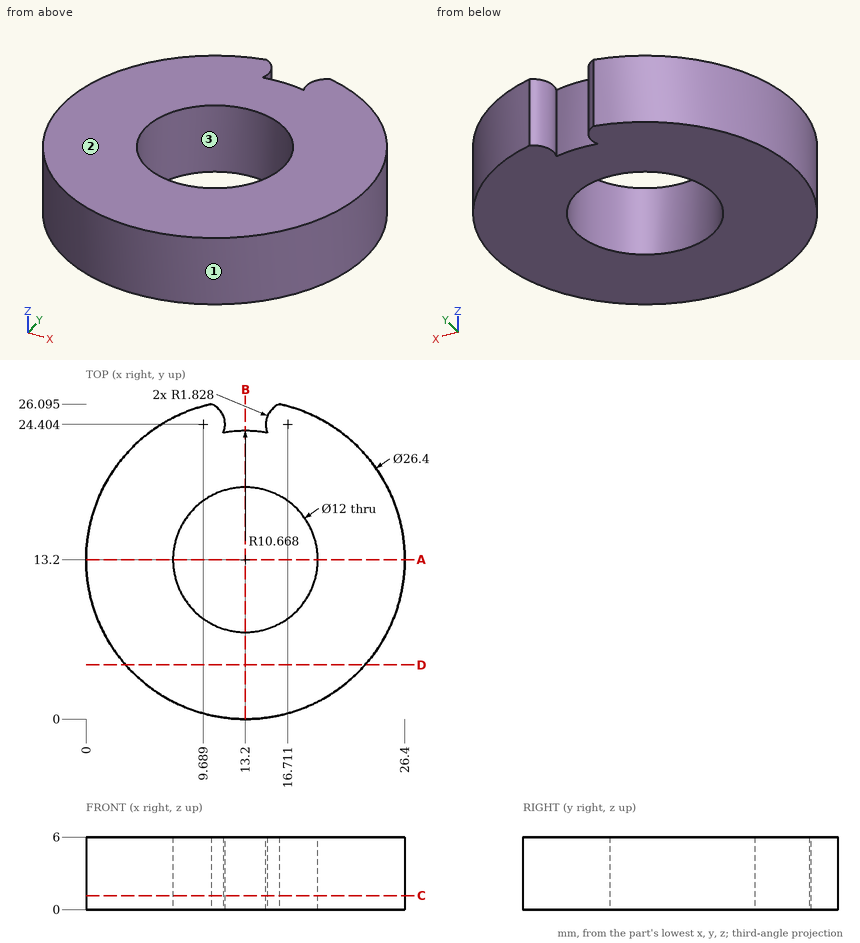
Here's the drawing with two shaded views (mm, measured from the low corner). I have some questions. Give positions to 0.01 mm unless a question says otherwise; leave off trailing zeros. Write each loop counter-clockwise with the first axis right and the second up, starting at its lowest first coordinate (ties: lowest second). Pieces come first, ordered by that corner, then holes. Notation, with made-up numbers: (41, 29) -> (71, 29) arc R19 cw to (71, 62) -> close; hole circle Ø6 at (-26, -1.75). An arc over 180 degrees is marked (long way). One line per item, written item: value.
Q1. Imagine slicing it at A-A on y = 13.2. Please give me the cut outline in (x, z).
Results found:
outline: (0, 0) -> (7.2, 0) -> (7.2, 6) -> (0, 6) -> close; (19.2, 0) -> (26.4, 0) -> (26.4, 6) -> (19.2, 6) -> close
Q2. For P1, Ø3, axis at y = 22.5, z = 4, coming from the +X side; P2, Ø1, axis at y = 3, z = 1.5, coming from the -X side; P3, Ø1.5, axis at x = 18, z = 1, coming from the +Y side, each with a flat end and sliding along its axis, tell me the tip position at first contact or that it passes through.
Results found:
P1: stops at x = 23.85
P2: stops at x = 4.25
P3: stops at y = 25.76
Q3. Imagine slicing it at D-D on y = 4.5. Please give me the cut outline in (x, z), and give its area (3 significant figures).
Results found:
outline: (3.27, 0) -> (23.13, 0) -> (23.13, 6) -> (3.27, 6) -> close
area: 119 mm^2
Q4. Imagine slicing it at B-B on x = 13.2. Please give me the cut outline in (y, z).
Results found:
outline: (0, 0) -> (7.2, 0) -> (7.2, 6) -> (0, 6) -> close; (19.2, 0) -> (23.87, 0) -> (23.87, 6) -> (19.2, 6) -> close
Q5. Please list where these lines run through material, in increasing order: line 1 (Y direction, x = 13.5, z = 3.3) (1 decimal); line 2 (X direction, y = 11, z = 2.35) (1 decimal); line 3 (X direction, y = 9, z = 0.3) (1 decimal). Write a range as [from, to].
Results found:
line 1: y = [0, 7.2], [19.2, 23.9]
line 2: x = [0.2, 7.6], [18.8, 26.2]
line 3: x = [0.7, 8.9], [17.5, 25.7]
Q6. We'd pull the mould along X, two halves only. Please class the marked faces 1, 2 and 3: +X half, -X half, draft (parallel to the pull), parting line (faces both ways), or undercut.
Results found:
face 1: parting line
face 2: draft
face 3: undercut
Q7. Imagine slicing it at C-C on z = 1.15. Please give me the cut outline in (x, y) (1 decimal).
Results found:
outline: (10.4, 26.1) arc R13.2 ccw (long way) to (16, 26.1) arc R1.8 ccw to (15, 23.7) arc R10.7 ccw to (11.4, 23.7) arc R1.8 ccw to start; hole circle Ø12 at (13.2, 13.2)
